Part print with two shaded views. Sizes in mm from the minimum x, y, z corner. A direction names the side the tool comes from. Round coordinates to 2 decimals unless told otherwise and drop trailing zeros. Write each loop counter-clockwise with the first axis right and the second up, starting at its lowest first coordinate (ties: lowest second). Pieces come first, ordered by that corner, then holes.
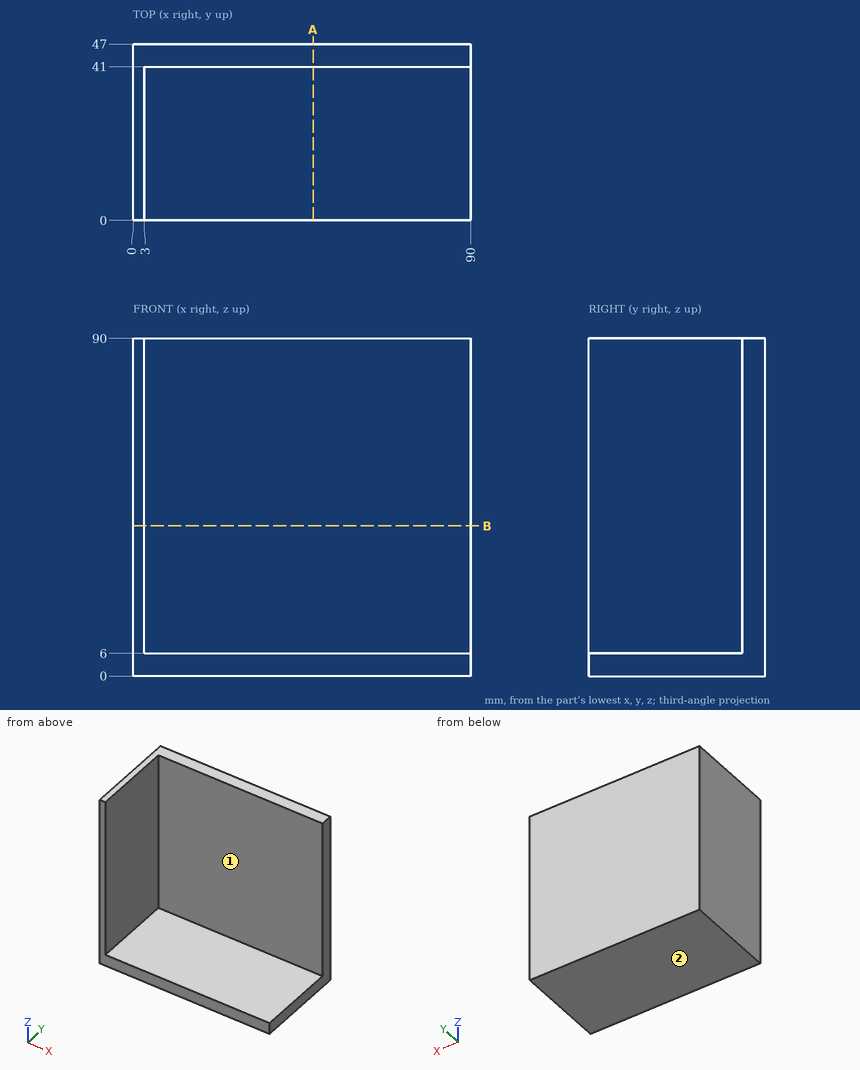
Q1. Which spindle directions (+Z, -Z, +X, -X, +Y, -Y) get a long thin tool onto all of the face, cutting with end or side? Do the marked faces 1 and 2. Say none if no direction does.
Values follow:
face 1: +Z, +X, -Y
face 2: -Z, +X, -X, +Y, -Y
Q2. Cut at A-A on x = 48. Write the cut outline in (y, z).
Values follow:
outline: (0, 0) - (47, 0) - (47, 90) - (41, 90) - (41, 6) - (0, 6) - close
Q3. Drop flat-ended pins along their axis: pin 1 (2 mm diameter, centred on y = 39.5, z = 15, fed in from +X); pin 2 (12.5 mm diameter, centred on x = 33.5, y = 11, fed in from +Z); pin 3 (12 mm diameter, centred on x = 74, z = 24, fed in from -Y). Give the stop position or say it passes through.
Values follow:
pin 1: stops at x = 3
pin 2: stops at z = 6
pin 3: stops at y = 41
Q4. Wall check: L1, parallel to Y at x = 50.5, z = 30; L2, parallel to Z at x = 64.5, y = 4; L3, parallel to X at y = 24.5, z = 34. Give the ranges that are in metal, low to high.
Values follow:
L1: y = 41 to 47
L2: z = 0 to 6
L3: x = 0 to 3
Q5. Cut at B-B on z = 40. Write the cut outline in (x, y).
Values follow:
outline: (0, 0) - (3, 0) - (3, 41) - (90, 41) - (90, 47) - (0, 47) - close
